```python
from build123d import *

# Parameters (mm, degrees)
SKETCH_1_R          = 25
EXTRUDE_1_DEPTH     = 30
CUT_EXTRUDE_1_DEPTH = 31.5
SKETCH_7_R          = 21
CUT_EXTRUDE_2_DEPTH = 7
SKETCH_8_R          = 21
CUT_EXTRUDE_3_DEPTH = 3.5
SKETCH_9_R          = 18
CUT_EXTRUDE_4_DEPTH = 107.5


with BuildPart() as part:
    # 草图1 → 凸台-拉伸1 (new body)
    with BuildSketch(Plane(origin=(0, 0, 0), x_dir=(1, 0, 0), z_dir=(0, 1, 0))):
        Circle(SKETCH_1_R)
    extrude(amount=EXTRUDE_1_DEPTH)

    # 草图3 → 切除-拉伸1 (cut, symmetric)
    with BuildSketch(Plane(origin=(0, 0, 0), x_dir=(0, 0, -1), z_dir=(1, 0, 0))):
        Polygon((-25, 18), (25, 25.188898505), (25, 39.510034579), (-25, 39.510034579), align=None)
        Polygon((25, 0), (-25, 7.188898505), (-25, -17.358468242), (25, -17.358468242), align=None)
    extrude(amount=CUT_EXTRUDE_1_DEPTH, both=True, mode=Mode.SUBTRACT)

    # 草图7 → 切除-拉伸2 (cut)
    with BuildSketch(Plane(origin=(0, 21.15708772, 3.041923126), x_dir=(1, 0, 0), z_dir=(0, 0.989821487, 0.142314524))):
        with Locations((0, 3.07320377)):
            Circle(SKETCH_7_R)
    extrude(amount=-CUT_EXTRUDE_2_DEPTH, mode=Mode.SUBTRACT)

    # 草图8 → 切除-拉伸3 (cut)
    with BuildSketch(Plane(origin=(0, 3.521649349, -0.506335595), x_dir=(-1, 0, 0), z_dir=(0, -0.989821487, 0.142314524))):
        with Locations((0, 0.488457665)):
            Circle(SKETCH_8_R)
    extrude(amount=-CUT_EXTRUDE_3_DEPTH, mode=Mode.SUBTRACT)

    # 草图9 → 切除-拉伸4 (cut)
    with BuildSketch(Plane(origin=(0, 0, 0), x_dir=(1, 0, 0), z_dir=(0, 1, 0))):
        Circle(SKETCH_9_R)
    extrude(amount=CUT_EXTRUDE_4_DEPTH, mode=Mode.SUBTRACT)


solid = part.part
```
Work out the finished part from the listing and answer in its coordinate system (mm). A direction names the side the tool comes from. Coordinates: 2 decimals unless noted, no trailing zeros. Loops run counter-clockwise (first coordinate to the right, second up) from the corner with the lowest first, then second, coordinate; pieces in that order, holes last. Notation, with made-up numbers: (8.5, 0.5) - (39.5, 0.5) arc R16 ccw to (39.5, 8.5) - close; hole circle Ø7 at (32, 62). An arc over 180 degrees is marked (long way). Use a Markdown table: item, result.
Item 1: The mould has two halves that part along Y. Classify faces 3 (the cylindrical face through (4.552, 8.078, 19.057)), 4 (the flat face through (0.117, 6.506, 20.254)), 5 (the flat face through (16.55, 19.714, 13.08)): +Y half, -Y half, draft (parallel to the pull), parting line (faces both ways), or undercut.
Evaluation:
| item | result |
|---|---|
| face 3 | undercut |
| face 4 | -Y half |
| face 5 | +Y half |
Item 2: Find section C-C, the plane x = -8. Determine the outline of the cut face in (y, z), and give its area (3 significant figures).
Evaluation:
| item | result |
|---|---|
| outline | (0.19, -23.69) - (25, -23.69) - (24.36, -19.22) - (17.43, -20.22) - (16.84, -16.12) - (4.81, -16.12) - (4.15, -20.71) - (0.69, -20.21) - close; (6.22, 18.23) - (9.68, 17.73) - (9.45, 16.12) - (12.2, 16.12) - (11.9, 18.22) - (18.83, 19.22) - (18.19, 23.69) - (7, 23.69) - close |
| area | 207 mm2 |
Item 3: Given pin 1 Ø3 at (x, z) = (14, -11.5) entering from +Y; pin 2 Ø8 at (x, z) = (18, 10) entering from +Y; pin 3 Ø6 at (x, y) = (-12, 6.5) entering from +Z, each flat-ended and moving along its own axis, determine where each tip first touches the part or whether it passes through.
Evaluation:
| item | result |
|---|---|
| pin 1 | stops at y = 16.39 |
| pin 2 | stops at y = 20.66 |
| pin 3 | stops at z = 23.31 |
Item 4: Find section A-A, the plane x = -2. Determine the outline of the cut face in (y, z).
Evaluation:
| item | result |
|---|---|
| outline | (0.01, -24.92) - (25.18, -24.92) - (24.57, -20.69) - (17.64, -21.69) - (17.09, -17.89) - (4.56, -17.89) - (3.94, -22.18) - (0.48, -21.68) - close; (6.43, 19.7) - (9.89, 19.2) - (9.7, 17.89) - (11.95, 17.89) - (11.69, 19.7) - (18.62, 20.69) - (18.01, 24.92) - (7.18, 24.92) - close |
Item 5: For faces 1 (the flat face through (-4.765, 17.115, -18.03)), 2 (the cylindrical face through (-2.343, 10.707, -17.847)), determine the directions among +Z, -Z, +X, -X, +Y, -Y from which every point of the face is accessible in a straight line to the end or side of a thin tool.
Evaluation:
| item | result |
|---|---|
| face 1 | none |
| face 2 | +Y, -Y |
Item 6: Find section B-B, the plane x = -19. Determine the outline of the cut face in (y, z).
Evaluation:
| item | result |
|---|---|
| outline | (1.26, -16.25) - (23.93, -16.25) - (22.87, -8.85) - (15.94, -9.85) - (13.39, 7.86) - (20.32, 8.85) - (19.26, 16.25) - (5.93, 16.25) - (4.73, 7.86) - (8.19, 7.37) - (5.64, -10.34) - (2.18, -9.84) - close |
Item 7: Consider probe 1 along X at (y, z) = (9.5, 0); probe 2 along X at (y, z) = (18, 11); probe 3 along Z at (x, y) = (0, 14). Determine where each line is inside the solid, lowest interval first. Write a range as from..to.
Evaluation:
| item | result |
|---|---|
| probe 1 | x = -25..-18, 18..25 |
| probe 2 | x = -22.45..-17.64, 17.64..22.45 |
| probe 3 | z = -25..-18, 20.12..25 |
